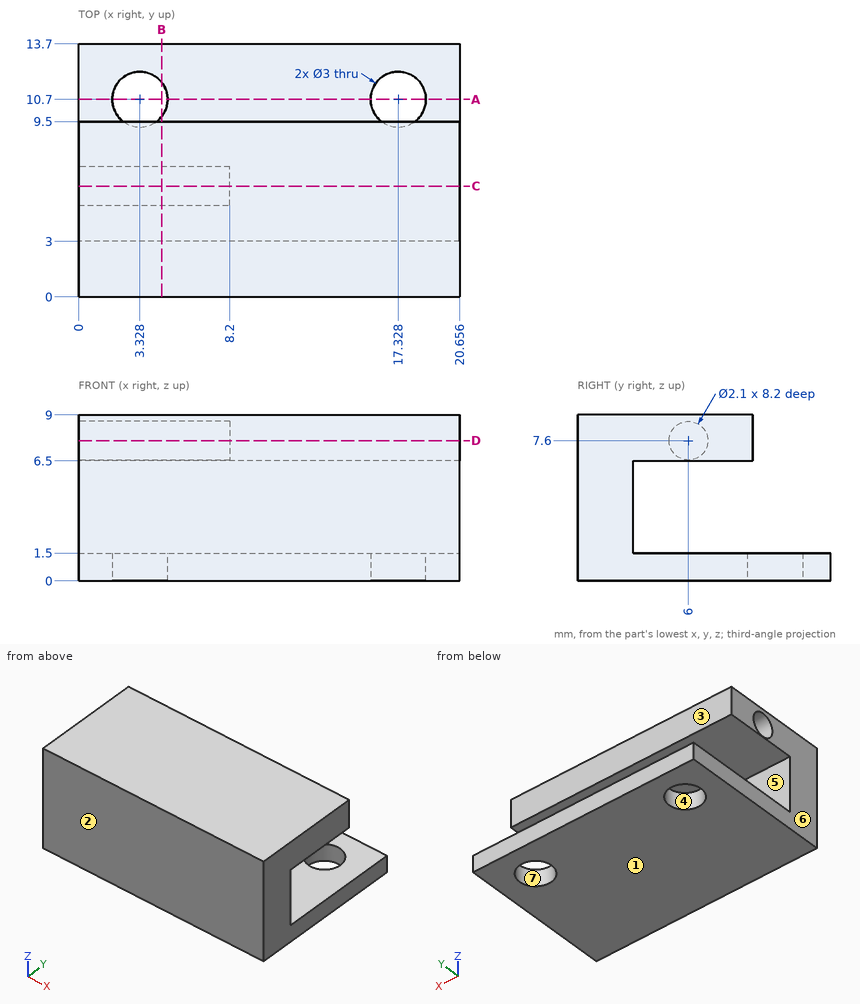
Job drawing, mm, ordinate dimensions from the low corner. One solid piece. A direction names the side the tool comes from. Give positions to 0.01 mm unless a question says otherwise; leave off trailing zeros. Order: outer loops, then holes, each group sorted by start corner. A loop starts at its lowest first (then second) coordinate and runs counter-clockwise, first axis right, second up. Notation, with made-up numbers: (-40, -16.5) - (7, -16.5) arc R10 ccw to (7, 2.5) - close; hole circle Ø6 at (52.5, 65). An arc over 180 degrees is marked (long way). One line per question, with ' | ' between items.
1. Band-saw the part on A-A on y = 10.7. List the corners of the cut face in (x, z).
Filled in:
outline: (0, 0) - (1.83, 0) - (1.83, 1.5) - (0, 1.5) - close; (4.83, 0) - (15.83, 0) - (15.83, 1.5) - (4.83, 1.5) - close; (18.83, 0) - (20.66, 0) - (20.66, 1.5) - (18.83, 1.5) - close
2. Which spindle directions (+Z, -Z, +X, -X, +Y, -Y) get a long thin tool onto all of the face, cutting with end or side? Do the marked faces 5, 6 and 7. Say none if no direction does.
Filled in:
face 5: +X, -X, +Y | face 6: +Z, -Z, -X, +Y, -Y | face 7: -Z
3. Drill centre lines: probe 1 along X at (y, z) = (10.7, 0.5); probe 2 along Z at (x, y) = (1.25, 4.5); probe 3 along X at (y, z) = (9.5, 0.5) (1 decimal). Where is each one in solid material? Low to high.
Filled in:
probe 1: 0 to 1.83, 4.83 to 15.83, 18.83 to 20.66 | probe 2: 0 to 1.5, 6.5 to 9 | probe 3: 0 to 2.4, 4.2 to 16.4, 18.2 to 20.7
4. Band-saw the part on B-B on x = 4.5. List the corners of the cut face in (y, z).
Filled in:
outline: (0, 0) - (9.76, 0) - (9.76, 1.5) - (3, 1.5) - (3, 6.5) - (9.5, 6.5) - (9.5, 9) - (0, 9) - close; (11.64, 0) - (13.7, 0) - (13.7, 1.5) - (11.64, 1.5) - close; hole circle Ø2.1 at (6, 7.6)
5. Band-saw the part on D-D on z = 7.6. List the corners of the cut face in (x, y), then the cut area to 3 significant figures.
Filled in:
outline: (0, 0) - (20.66, 0) - (20.66, 9.5) - (0, 9.5) - (0, 7.05) - (8.2, 7.05) - (8.2, 4.95) - (0, 4.95) - close | area: 179 mm²
6. Pull direction Y, two halves, no side cores. Call the marked faces 1, 2, 3 and 4: +Y half, -Y half, draft (parallel to the pull), parting line (faces both ways), or undercut.
Filled in:
face 1: draft | face 2: -Y half | face 3: +Y half | face 4: undercut
7. Drop flat-ended pins along their axis: P1, Ø2, axis at x = 5, z = 6.5, coming from the +Y side; P2, Ø1, axis at y = 9.5, z = 3, coming from the +X side. Give the stop position or say it passes through.
Filled in:
P1: y = 9.5 | P2: through
8. Band-saw the part on C-C on y = 6. List the corners of the cut face in (x, z).
Filled in:
outline: (0, 0) - (20.66, 0) - (20.66, 1.5) - (0, 1.5) - close; (0, 6.5) - (20.66, 6.5) - (20.66, 9) - (0, 9) - (0, 8.65) - (8.2, 8.65) - (8.2, 6.55) - (0, 6.55) - close
